from build123d import *

# Parameters (mm, degrees)
F1_DEPTH = 3
F2_W     = 10.790673
F2_H     = 8
F2_W_2   = 11.792415
F2_H_2   = 10
F2_W_3   = 13.604847
F2_H_3   = 13
F2_W_4   = 18.819063
F2_H_4   = 16
F3_DEPTH = 25
F4_R     = 5
F5_R     = 3
F6_R     = 5
F7_R     = 5
F8_R     = 5
F9_R     = 5
F10_R    = 5
F11_R    = 5


with BuildPart() as f1:
    # F0 (on Front) → F1 (new body)
    with BuildSketch(Plane.XZ):
        Polygon((15, 75), (-15, 75), (-15, 11.736112), (-8.253973, 0), (-8.253973, -75), (0, -75), (8.253973, -75), (8.253973, 0), (15, 11.736112), align=None)
    extrude(amount=F1_DEPTH)

    # F2 (on face) → F3 (cut)
    with BuildSketch(Plane.XZ.offset(3)):
        Polygon((-8.118863, 71.253784), (-15, 71.253784), (-17.755223, 71.253784), (-17.755223, 65.253784), (-8.118863, 65.253784), align=None)
        with Locations((-12.433694, 59.144969)):
            Rectangle(F2_W, F2_H)
        with Locations((-12.069519, 45.514927)):
            Rectangle(F2_W_2, F2_H_2)
        with Locations((-12.249198, 29.82161)):
            Rectangle(F2_W_3, F2_H_3)
        with Locations((14.454825, 59.229082)):
            Rectangle(F2_W_4, F2_H_4)
    extrude(amount=-F3_DEPTH, mode=Mode.SUBTRACT)

    # F4
    f4_edges = [f1.edges().sort_by_distance(p)[0] for p in [
        (15, -1.5, 75),
    ]]
    fillet(f4_edges, radius=F4_R)

    # F5
    f5_edges = [f1.edges().sort_by_distance(p)[0] for p in [
        (-15, -1.5, 75),
    ]]
    fillet(f5_edges, radius=F5_R)

    # F6
    f6_edges = [f1.edges().sort_by_distance(p)[0] for p in [
        (15, -1.5, 11.736112),
    ]]
    fillet(f6_edges, radius=F6_R)

    # F7
    f7_edges = [f1.edges().sort_by_distance(p)[0] for p in [
        (8.253973, -1.5, 0),
    ]]
    fillet(f7_edges, radius=F7_R)

    # F8
    f8_edges = [f1.edges().sort_by_distance(p)[0] for p in [
        (-15, -1.5, 11.736112),
    ]]
    fillet(f8_edges, radius=F8_R)

    # F9
    f9_edges = [f1.edges().sort_by_distance(p)[0] for p in [
        (-8.253973, -1.5, 0),
    ]]
    fillet(f9_edges, radius=F9_R)

    # F10
    f10_edges = [f1.edges().sort_by_distance(p)[0] for p in [
        (-8.253973, -1.5, -75),
    ]]
    fillet(f10_edges, radius=F10_R)

    # F11
    f11_edges = [f1.edges().sort_by_distance(p)[0] for p in [
        (8.253973, -1.5, -75),
    ]]
    fillet(f11_edges, radius=F11_R)


solid = f1.part
Model file for the job. Use its own axes, mm. A direction names the side the tool comes from. Coordinates: 2 decimals unless noted, no trailing zeros. Write each loop counter-clockwise with the first axis right and the second up, starting at its lowest first coordinate (ties: lowest second). Pieces come first, ordered by that corner, then holes. Notation, with made-up numbers: (49.25, -32) - (98.25, -32) arc R26 cw to (98.25, 0) - close; hole circle Ø10 at (30, -2.5). An arc over 180 degrees is marked (long way). Write each question's results on one line, items separated by ' | '. Start each with the question number.
1) 3-axis set-ups, long thin cutter, end or side, ignore diameter. For faces 1 (the face through (-11, -2, 40.515)), 2 (the face through (10, -2, 67.229)), 3 (the face through (-6.828, -1.521, -73.496)): which of +Z, -Z, +X, -X, +Y, -Y reach the whole face in a straight line?
2) Cut at B-B (z = 28). Write the cut outline in (x, y), then the cut area to 3 significant figures.
3) Cut at A-A (x = 7). Write the cut outline in (y, z), then the cut area to 3 significant figures.
4) Probe line 1 along Z through (x, y) = (-8.75, -0.8); line 2 along Z through (x, y) = (-11.5, -2.1); line 3 along X through (y, z) = (-1.35, 56). List the from-to ranges inside material, lowest first. Write a range as from..to.
5) Mould opens along Z. For faces 4 (the face through (-10, -2, 36.322)), 5 (the face through (-8.254, -1, -35)), 6 (the face through (14.836, -1.521, 11.799)) say: pulls with the +Z half, pulls with the -Z half, needs draft (parallel to the pull), parting line crosses it, or undercut.
6) Cut at C-C (z = 43). Write the cut outline in (x, y), then the cut area to 3 significant figures.
7) Flat gauge pins, fed straight in: P1, Ø1, axis at y = -1, z = -5, coming from the -X side; P2, Ø1, axis at x = -9.5, z = 1, coming from the +Y side; P3, Ø0.9, axis at x = -10.5, y = -1.5, coming from the -Z side; P4, Ø1.5, axis at y = -1, z = 31, coming from the -X side. Where does each tip first touch, or does it go through?
Returned:
1) face 1: -X, +Y, -Y | face 2: +X, +Y, -Y | face 3: -Z, -X, +Y, -Y
2) outline: (-5.45, -3) - (15, -3) - (15, 0) - (-5.45, 0) - close | area: 61.3 mm^2
3) outline: (-3, -73.31) - (0, -73.31) - (0, 51.23) - (-3, 51.23) - close; (-3, 67.23) - (0, 67.23) - (0, 75) - (-3, 75) - close | area: 397 mm^2
4) line 1: 0.84..23.32, 36.32..40.51, 50.51..55.14, 63.14..65.25, 71.25..75 | line 2: 5.65..23.32, 36.32..40.51, 50.51..55.14, 63.14..65.25, 71.25..75 | line 3: -7.04..5.05
5) face 4: undercut | face 5: needs draft | face 6: pulls with the -Z half
6) outline: (-6.17, -3) - (15, -3) - (15, 0) - (-6.17, 0) - close | area: 63.5 mm^2
7) P1: x = -8.25 | P2: through | P3: z = 3.12 | P4: x = -5.45
